from build123d import *

# Parameters (mm, degrees)
F0_W     = 40
F0_H     = 40
F0_W_2   = 35
F0_H_2   = 35
F1_DEPTH = 730
F2_R     = 6
F3_DEPTH = 5


with BuildPart() as f1:
    # F0 (on Right) → F1 (new body, symmetric)
    with BuildSketch(Plane.YZ):
        Rectangle(F0_W, F0_H)
        Rectangle(F0_W_2, F0_H_2, mode=Mode.SUBTRACT)
    extrude(amount=F1_DEPTH, both=True)

    # F2 (on face) → F3 (join)
    with BuildSketch(Plane.YZ.offset(730)):
        with BuildLine():
            Line((20, -20), (20, 20))
            Line((20, 20), (-20, 20))
            Line((-20, 20), (-20, -57))
            ThreePointArc((-20, -57), (-19.1213203436, -59.1213203436), (-17, -60))
            Line((-17, -60), (17, -60))
            ThreePointArc((17, -60), (19.1213203436, -59.1213203436), (20, -57))
            Line((20, -57), (20, -20))
        make_face()
        with Locations((0, -40)):
            Circle(F2_R, mode=Mode.SUBTRACT)
    extrude(amount=F3_DEPTH)

    # F4: F1 across plane


with BuildPart() as f1_1:
    add(f1.part)
    add(f1.part.mirror(Plane.YZ))


solid = f1_1.part
Can you work these out from the model? Positions are in its coordinate system, mm. A direction names the side the tool comes from. Round coordinates to 2 decimals unless told otherwise and drop trailing zeros. Order: outer loops, then holes, each group sorted by start corner. A loop starts at its lowest first (then second) coordinate and runs counter-clockwise, first axis right, second up. Notation, with made-up numbers: (58, -0.75) -> (63, -0.75) arc R4 ccw to (63, 5.25) -> close; hole circle Ø6 at (32, 68.5). An arc over 180 degrees is marked (long way). Write each question's results on one line, items separated by ' | '. Start each with the question number.
Item 1: Which directions (+Z, -Z, +X, -X, +Y, -Y) give clear straight access to the entire face, cutting with the end or side of a thin tool? Please do faces 1 (the flat face through (10, 0, -17.5)), 2 (the flat face through (730, -5, -35)), 3 (the flat face through (10, -20, -1)).
Item 2: If we section it at B-B, the plane x = 269: Write out the boundary of the cut face in (y, z).
Item 3: Will these pins go through, and if not, where does the flat tip stop? pin 1 (9.5 mm diameter, centred on y = 0, z = -40, fed in from -X); pin 2 (5 mm diameter, centred on x = -94, y = 0, fed in from -Z).
Item 4: Please list where these lines run through material, in increasing order: L1, parallel to X at y = 9, z = 11; L2, parallel to Z at x = -733, y = 0; L3, parallel to Z at x = 263, y = 7.5.
Item 5: If we section it at A-A, the plane y = 0: Write out the boundary of the cut face in (x, z).
Item 6: Thinking about a two-plate mould opening in X: for faces 4 (the flat face through (735, 0, -19)), 5 (the flat face through (10, 20, -2)), 6 (the flat face through (10, -17.5, 0)), which applies, +X half, -X half, draft (parallel to the pull), parting line (faces both ways), or undercut?
Results:
1) face 1: none | face 2: -Z, +Y, -Y | face 3: +Z, -Z, +X, -X, -Y
2) outline: (-20, -20) -> (20, -20) -> (20, 20) -> (-20, 20) -> close; hole (-17.5, -17.5) -> (17.5, -17.5) -> (17.5, 17.5) -> (-17.5, 17.5) -> close
3) pin 1: passes through | pin 2: stops at z = -20
4) L1: x = -735 to -730, 730 to 735 | L2: z = -60 to -46, -34 to 20 | L3: z = -20 to -17.5, 17.5 to 20
5) outline: (-735, -60) -> (-730, -60) -> (-730, -46) -> (-735, -46) -> close; (-735, -34) -> (-730, -34) -> (-730, -20) -> (730, -20) -> (730, -34) -> (735, -34) -> (735, 20) -> (-735, 20) -> close; (730, -60) -> (735, -60) -> (735, -46) -> (730, -46) -> close; hole (-730, -17.5) -> (730, -17.5) -> (730, 17.5) -> (-730, 17.5) -> close
6) face 4: +X half | face 5: draft | face 6: undercut
